Design review of the part shown in the three views and the two pictorial views. Dimensions are in mm from the part's minimum x, y and z. A direction names the side the tool comes from. Give positions to 0.01 mm unless a question says otherwise; leave off trailing zeros. Loops run counter-clockwise (first coordinate to the right, second up) from the corner with the lowest first, then second, coordinate; pieces in that order, holes last. Notation, with made-up numbers: (78.25, -28.75) - (106.25, -28.75) arc R11 cw to (106.25, -22.75) - close; hole circle Ø11 at (-3.5, 42.5). An arc over 180 degrees is marked (long way). Answer as a JSON object with one key per item and string values.
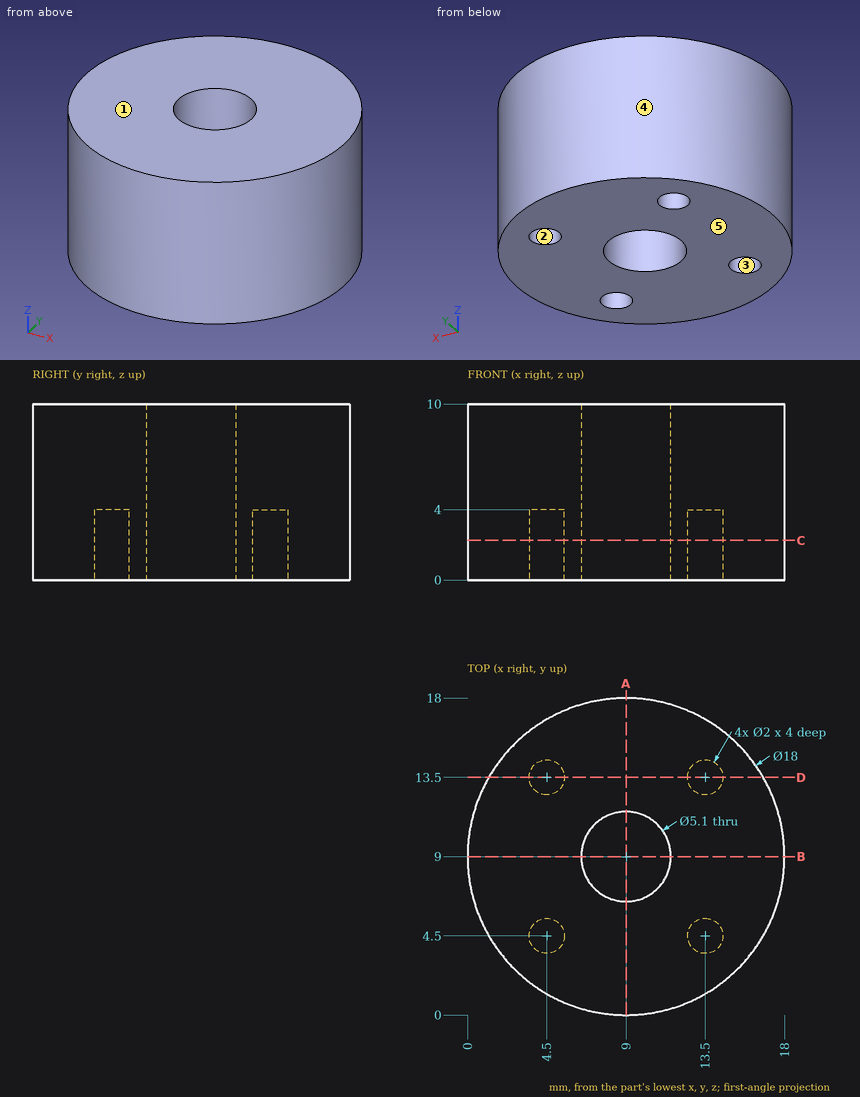
Q1. Consider section C-C, the plane z = 2.25. State the section outline as (x, y) points.
Results:
{"outline": "circle Ø18 at (9, 9); hole circle Ø2 at (4.5, 4.5); hole circle Ø2 at (4.5, 13.5); hole circle Ø5.1 at (9, 9); hole circle Ø2 at (13.5, 4.5); hole circle Ø2 at (13.5, 13.5)"}
Q2. Clearance check with flat-ended pins moving along their axes: pin 1 Ø0.6 at (x, y) = (4.5, 4.5) entering from -Z; pin 2 Ø4 at (x, z) = (3, 6.5) entering from +Y; pin 3 Ø6 at (y, z) = (4.5, 4) entering from +X. State where each tip first meets the part, or that it passes through.
Results:
{"pin 1": "stops at z = 4", "pin 2": "stops at y = 17.06", "pin 3": "stops at x = 17.87"}
Q3. The part is to be moulded in two halves that separate along Y. For the marked faces 3, 4 and 5, say which applies: +Y half, -Y half, draft (parallel to the pull), parting line (faces both ways), or undercut.
Results:
{"face 3": "undercut", "face 4": "parting line", "face 5": "draft"}
Q4. Consider section D-D, the plane y = 13.5. State the section outline as (x, z) points.
Results:
{"outline": "(1.21, 0) - (3.5, 0) - (3.5, 4) - (5.5, 4) - (5.5, 0) - (12.5, 0) - (12.5, 4) - (14.5, 4) - (14.5, 0) - (16.79, 0) - (16.79, 10) - (1.21, 10) - close"}
Q5. To check wall thickness, follow probe 1 along X at (y, z) = (4.5, 2.3); probe 2 along Y at (x, z) = (9, 5.5); probe 3 along Y at (x, z) = (7.5, 1). State the ranges of each line that lie inside material, in increasing order. Write a range as [from, to].
Results:
{"probe 1": "x = [1.21, 3.5], [5.5, 12.5], [14.5, 16.79]", "probe 2": "y = [0, 6.45], [11.55, 18]", "probe 3": "y = [0.13, 6.94], [11.06, 17.87]"}
Q6. For the marked faces 1 and 2, list the 3-axis set-ups (+Z, -Z, +X, -X, +Y, -Y) from which the entire face can be reached by the end or side of a thin tool; tool diameter is ignored.
Results:
{"face 1": "+Z, +X, -X, +Y, -Y", "face 2": "-Z"}
Q7. Consider section A-A, the plane x = 9. State the section outline as (y, z) points.
Results:
{"outline": "(0, 0) - (6.45, 0) - (6.45, 10) - (0, 10) - close; (11.55, 0) - (18, 0) - (18, 10) - (11.55, 10) - close"}
